CAD build for the part. Positions are in the model's coordinates, mm. Face numbers are marked on the shaded views. A direction names the side the tool comes from. Coordinates: 2 decimals unless noted, no trailing zeros. Order: outer loops, then holes, each group sorted by start corner. A loop starts at its lowest first (then second) coordinate and runs counter-clockwise, first axis right, second up. Notation, with made-up numbers: M -22.75,34.25 L -8.75,34.25 A32 cw -8.75,66.25 Z; hole C 68,13.5 d10. An arc over 180 degrees is marked long. Write item = value, one per line.
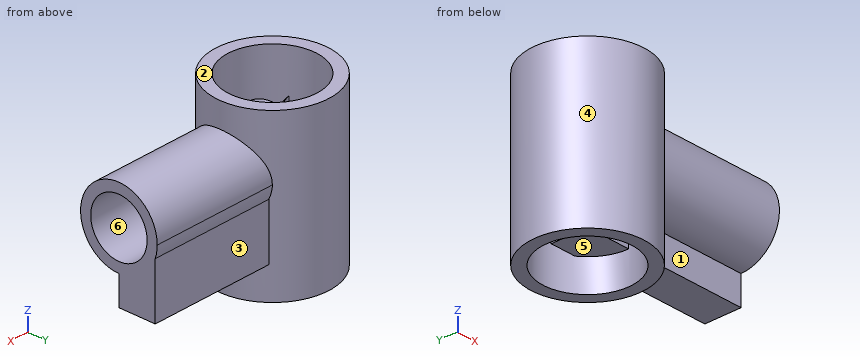
from build123d import *

# Parameters (mm, degrees)
F0_R     = 68.9306074925
F0_R_2   = 54.2522801739
F1_DEPTH = 196.7971026897
F3_DEPTH = 202.3541331291
F4_R     = 34.4816495033
F5_DEPTH = 250.7874369621


with BuildPart() as f1:
    # F0 (on Top) → F1 (new body)
    with BuildSketch(Plane.XY):
        Circle(F0_R)
        Circle(F0_R_2, mode=Mode.SUBTRACT)
    extrude(amount=F1_DEPTH)

    # F2 (on Right) → F3 (join)
    with BuildSketch(Plane.YZ):
        with BuildLine():
            Line((0, 73.7437401834), (0, 120.5569505692))
            Line((0, 120.5569505692), (44.4016605616, 120.5569505692))
            Line((44.4016605616, 120.5569505692), (44.4016605616, 105.725591697))
            ThreePointArc((44.4016605616, 105.725591697), (46.2063899475, 113.043882312), (46.8132103857, 120.5569505692))
            ThreePointArc((46.8132103857, 120.5569505692), (-33.1019385129, 153.658889082), (0, 73.7437401834))
        make_face()
        with BuildLine():
            Line((44.4016605616, 120.5569505692), (0, 120.5569505692))
            Line((0, 120.5569505692), (0, 73.7437401834))
            ThreePointArc((0, 73.7437401834), (27.3603101539, 82.5715573909), (44.4016605616, 105.725591697))
            Line((44.4016605616, 105.725591697), (44.4016605616, 120.5569505692))
        make_face()
        with BuildLine():
            ThreePointArc((44.4016605616, 105.725591697), (27.3603101539, 82.5715573909), (0, 73.7437401834))
            Line((0, 73.7437401834), (0, 38.8107895851))
            Line((0, 38.8107895851), (44.4016605616, 38.8107895851))
            Line((44.4016605616, 38.8107895851), (44.4016605616, 105.725591697))
        make_face()
    extrude(amount=F3_DEPTH)

    # F4 (on face) → F5 (cut)
    with BuildSketch(Plane.YZ.offset(202.3541331291)):
        with Locations((0, 120.5569505692)):
            Circle(F4_R)
    extrude(amount=-F5_DEPTH, mode=Mode.SUBTRACT)


solid = f1.part
(1) Pull direction X, two halves, no side cores. Call the marked faces 4, 5 and 6: +X half, -X half, draft (parallel to the pull), parting line (faces both ways), or undercut.
Evaluation:
face_4 = parting line
face_5 = undercut
face_6 = draft
(2) Slice it at C-C, the plane z = 48. Write the cut outline in (x, y).
Evaluation:
outline = M 52.72,44.4 A68.93 ccw long 68.93,0 L 202.35,0 L 202.35,44.4 Z; hole M 0,0 L 0,44.4 L 31.17,44.4 A54.25 ccw long 54.25,0 Z
(3) Slice it at B-B, the plane y = 50. Write the cut outline in (x, z), then the cut area to 3 significant figures.
Evaluation:
outline = M -47.45,0 L -21.05,0 L -21.05,196.8 L -47.45,196.8 Z; M 21.05,0 L 47.45,0 L 47.45,196.8 L 21.05,196.8 Z
area = 10,400 mm²
(4) Wall check: line 1 (Z direction, x = 63, y = 0); line 2 (Z direction, x = 99.5, y = 7); line 3 (Y direction, x = 100, z = 69). Give the ranges that are in metal, low to high. Write a range as from..to.
Evaluation:
line_1 = 0..86.08, 155.04..196.8
line_2 = 38.81..86.79, 154.32..166.84
line_3 = 0..44.4
(5) Slice it at D-D, the plane y = -27.5. Write the cut outline in (x, z), then the cut area to 3 significant figures.
Evaluation:
outline = M -63.21,0 L -46.77,0 L -46.77,99.75 L -48.43,99.75 L -48.43,141.36 L -46.77,141.36 L -46.77,196.8 L -63.21,196.8 Z; M 0,82.67 L 46.77,82.67 L 46.77,0 L 63.21,0 L 63.21,82.67 L 202.35,82.67 L 202.35,99.75 L 0,99.75 Z; M 0,141.36 L 202.35,141.36 L 202.35,158.44 L 63.21,158.44 L 63.21,196.8 L 46.77,196.8 L 46.77,158.44 L 0,158.44 Z
area = 12,100 mm²
(6) Slice it at A-A, the plane x = -35.5. Write the cut outline in (y, z).
Evaluation:
outline = M -59.09,0 L -41.03,0 L -41.03,196.8 L -59.09,196.8 Z; M 41.03,0 L 59.09,0 L 59.09,196.8 L 41.03,196.8 Z
(7) Pin check, flat tips, straight feed: pin 1 Ø12 at (x, z) = (119, 35.5) entering from +Y; pin 2 Ø5 at (y, z) = (-28, 132.5) entering from +X; pin 3 Ø4 at (x, z) = (126, 92) entering from -Y. Stop position of each tip, or through.
Evaluation:
pin_1 = 44.4
pin_2 = -48.43
pin_3 = -38.55
(8) Tool access for the marked faces 1, 2 and 3: list every direction of +Z, -Z, +X, -X, +Y, -Y with a clear straight run to the whole face (end or side of a thin tool).
Evaluation:
face_1 = -Z, +X, -Y
face_2 = +Z, +X, -X, +Y, -Y
face_3 = -Z, +X, +Y
